Model file for the job. Use its own axes, mm. Face numbers are marked on the shaded views. A direction names the side the tool comes from. Give positions to 0.01 mm unless a question says otherwise; leave off trailing zeros. Loops run counter-clockwise (first coordinate to the right, second up) from the corner with the lowest first, then second, coordinate; pieces in that order, holes last. Notation, with made-up numbers: M 67,-29 L 118,-29 A37 cw 118,8 Z; hole C 62,69 d8. An arc over 180 degrees is marked long. Use CSV: the item, a comma, the result in double quotes. Start each with the question number.
(1) Tool access for the marked faces 1 and 2: list every direction of +Z, -Z, +X, -X, +Y, -Y with a clear straight run to the whole face (end or side of a thin tool).
(2) Slice it at A-A on z = 64.25. List the corners of the cut face in (x, y).
(3) Wall check: line 1 along X through (y, z) = (1.35, 9.35); line 2 along X through (y, z) = (3.15, 9.35); line 3 along Z through (x, y) = (103.2, 2.4). Give the ranges that are in metal, low to high. Write a range as from..to.
(4) Slice it at C-C on x = 19. List the corners of the cut face in (y, z).
(5) Slice it at B-B on x = 103.2. List the corners of the cut face in (y, z).
(6) Slice it at D-D on z = 25. List the corners of the cut face in (x, y).
(7) Flat gauge pins, fed straight in: P1, Ø2, axis at x = 43, z = 64.5, coming from the -Y side; P2, Ø1, axis at x = 103, z = 65, coming from the -Y side; P3, Ø0.8, axis at x = 40.5, y = -0.5, coming from the +Z side. Where does each tip first touch, or does it go through?
```python
from build123d import *

# Parameters (mm, degrees)
EXTRUDE_1_DEPTH     = 9.5
SKETCH_2_5_W        = 4.5
SKETCH_2_5_H        = 14
SKETCH_2_5_H_2      = 4.5
EXTRUDE_5_DEPTH     = 1.5
SKETCH_2_6_R        = 1.25
EXTRUDE_6_DEPTH     = 1
SKETCH_2_7_R        = 1.65
CUT_EXTRUDE_1_DEPTH = 4
SKETCH_3_W          = 14.5
SKETCH_3_H          = 74.8
CUT_EXTRUDE_2_DEPTH = 1.5
SKETCH_2_R          = 3.6
SKETCH_2_W          = 3.5
SKETCH_2_H          = 5.5
EXTRUDE_7_DEPTH     = 5


with BuildPart() as part:
    # Sketch 1 → Extrude 1 (new body)
    with BuildSketch(Plane(origin=(0, 0, 0), x_dir=(1, 0, 0), z_dir=(0, 1, 0))):
        with BuildLine():
            Line((6, 0), (143.8, 0))
            ThreePointArc((143.8, 0), (148.042640687, -1.757359313), (149.8, -6))
            Line((149.8, -6), (149.8, -68.8))
            ThreePointArc((149.8, -68.8), (148.042640687, -73.042640687), (143.8, -74.8))
            Line((143.8, -74.8), (6, -74.8))
            ThreePointArc((6, -74.8), (1.757359313, -73.042640687), (0, -68.8))
            Line((0, -68.8), (0, -6))
            ThreePointArc((0, -6), (1.757359313, -1.757359313), (6, 0))
        make_face()
    extrude(amount=EXTRUDE_1_DEPTH)

    # Sketch 2_5 → Extrude 5 (add)
    with BuildSketch(Plane(origin=(0, 0, 0), x_dir=(-1, 0, 0), z_dir=(0, -1, 0))):
        with Locations((-40.85, -52.05)):
            Rectangle(SKETCH_2_5_W, SKETCH_2_5_H)
        with Locations((-43.05, -63.8)):
            Rectangle(SKETCH_2_5_W, SKETCH_2_5_H_2)
    extrude(amount=EXTRUDE_5_DEPTH)

    # Sketch 2_6 → Extrude 6 (add)
    with BuildSketch(Plane(origin=(0, 0, 0), x_dir=(-1, 0, 0), z_dir=(0, -1, 0))):
        with Locations(Location((-130.8, -5.6, 0), (0, 0, 90))):
            Circle(SKETCH_2_6_R)
        with Locations(Location((-131.1, -55.65, 0), (0, 0, 90))):
            Circle(SKETCH_2_6_R)
        with Locations(Location((-47.7, -4.85, 0), (0, 0, 90))):
            Circle(SKETCH_2_6_R)
        with Locations(Location((-48.1, -68.75, 0), (0, 0, 90))):
            Circle(SKETCH_2_6_R)
        with Locations(Location((-22.8, -70.3, 0), (0, 0, 90))):
            Circle(SKETCH_2_6_R)
        with Locations(Location((-5.05, -71.05, 0), (0, 0, 90))):
            Circle(SKETCH_2_6_R)
        with Locations(Location((-5.05, -3.25, 0), (0, 0, 90))):
            Circle(SKETCH_2_6_R)
    extrude(amount=EXTRUDE_6_DEPTH)

    # Sketch 2_7 → Cut-Extrude 1 (cut)
    with BuildSketch(Plane(origin=(0, 0, 0), x_dir=(-1, 0, 0), z_dir=(0, -1, 0))):
        with Locations(Location((-103.2, -9.35, 0), (0, 0, 90))):
            Circle(SKETCH_2_7_R)
        with Locations(Location((-103.2, -64.25, 0), (0, 0, 90))):
            Circle(SKETCH_2_7_R)
        with Locations(Location((-59.2, -64.25, 0), (0, 0, 90))):
            Circle(SKETCH_2_7_R)
        with Locations(Location((-59.2, -9.35, 0), (0, 0, 90))):
            Circle(SKETCH_2_7_R)
    extrude(amount=-CUT_EXTRUDE_1_DEPTH, mode=Mode.SUBTRACT)

    # Sketch 3 → Cut-Extrude 2 (cut)
    with BuildSketch(Plane(origin=(0, 0, 0), x_dir=(1, 0, 0), z_dir=(0, 1, 0))):
        with Locations((142.55, -37.4)):
            Rectangle(SKETCH_3_W, SKETCH_3_H)
    extrude(amount=CUT_EXTRUDE_2_DEPTH, mode=Mode.SUBTRACT)

    # Sketch 2 → Extrude 7 (add)
    with BuildSketch(Plane(origin=(0, 0, 0), x_dir=(-1, 0, 0), z_dir=(0, -1, 0))):
        with Locations(Location((-19, -37.4, 0), (0, 0, 90))):
            Circle(SKETCH_2_R)
        with Locations((-29.05, -37.4)):
            Rectangle(SKETCH_2_W, SKETCH_2_H)
    extrude(amount=EXTRUDE_7_DEPTH)


solid = part.part
```
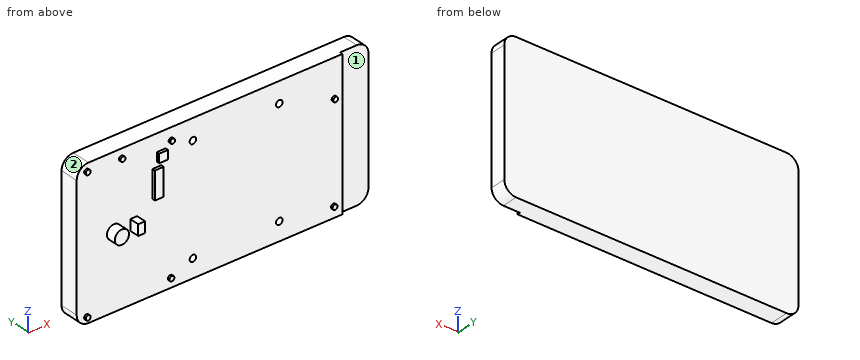
Reply:
1,face 1,"+Z, -Z, +X, -Y"
1,face 2,"+Z, -X, +Y, -Y"
2,outline,"M 0,0 L 40.8,0 L 40.8,-1.5 L 45.3,-1.5 L 45.3,0 L 57.55,0 L 57.55,4 L 60.85,4 L 60.85,0 L 101.55,0 L 101.55,4 L 104.85,4 L 104.85,0 L 135.3,0 L 135.3,1.5 L 149.8,1.5 L 149.8,9.5 L 0,9.5 Z"
3,line 1,"x = 0..57.55, 60.85..101.55, 104.85..135.3"
3,line 2,"x = 0..57.55, 60.85..101.55, 104.85..149.8"
3,line 3,"z = 0..7.7, 11..62.6, 65.9..74.8"
4,outline,"M -5,33.8 L 0,33.8 L 0,0 L 9.5,0 L 9.5,74.8 L 0,74.8 L 0,41 L -5,41 Z"
5,outline,"M 0,0 L 9.5,0 L 9.5,74.8 L 0,74.8 L 0,65.9 L 4,65.9 L 4,62.6 L 0,62.6 L 0,11 L 4,11 L 4,7.7 L 0,7.7 Z"
6,outline,"M 0,0 L 135.3,0 L 135.3,1.5 L 149.8,1.5 L 149.8,9.5 L 0,9.5 Z"
7,P1,"stops at y = -1.5"
7,P2,"stops at y = 4"
7,P3,"stops at z = 66.05"
